For this review, use the dimensioned drawing (mm, ordinates from the lowest corner) and the shaded views. Coordinates: 2 decimals unless noted, no trailing zeros. Loops run counter-clockwise (first coordinate to the right, second up) from the corner with the lowest first, then second, coordinate; pieces in that order, holes last. Notation, with made-up numbers: (13.5, 48.25) -> (23.5, 48.25) arc R14 ccw to (23.5, 72.25) -> close; hole circle Ø11 at (-34.5, 7.25). An arc over 180 degrees is marked (long way). Use one line per item in the form item = value. Start each with the question number.
1. Consider section B-B (z = 13.3). State the section outline as (x, y) points.
2. For pin 1 (0.8 mm diameter, centred on x = 3.5, y = 1, fed in from -Z); pin 2 (4 mm diameter, centred on x = 15, z = 21.3, fed in from -Y); pin 3 (0.5 mm diameter, centred on y = 1, z = 4, fed in from -X), all flat-tipped, find the tip position at first contact; note any pin that passes through.
3. Consider section D-D (x = 19.5). State the section outline as (y, z) points.
4. Consider section C-C (y = 0.7). State how many separate pieces and enclosed holes the cut face has, then the cut area to 3 significant figures.
5. Consider section A-A (x = 15). State the section outline as (y, z) points.
6. Wall thickness on line 1 (Z direction, x = 15, y = 0.5); line 2 (X direction, y = 1.35, z = 13.3); line 3 (X direction, y = 0.9, z = 21.3): over which ranges is each line inside the solid? List them lowest first. Write a range as from..to.
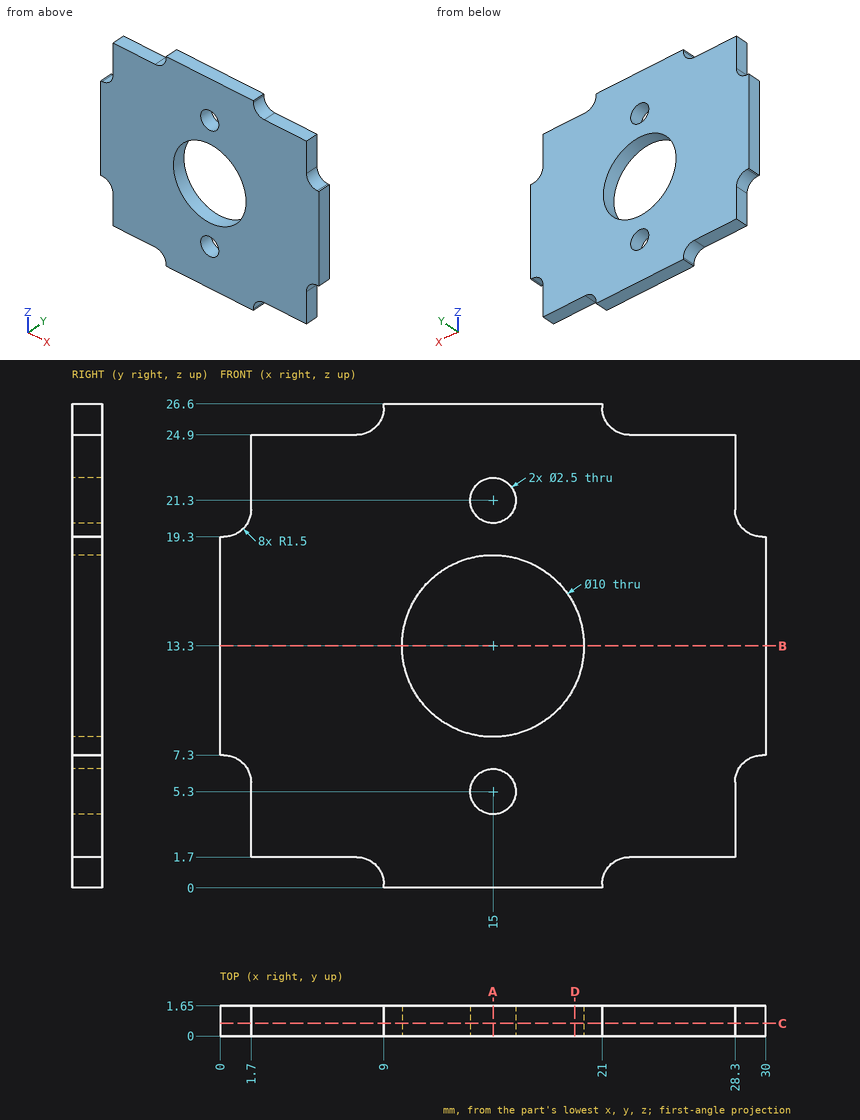
Geometry check:
q1.outline = (0, 0) -> (10, 0) -> (10, 1.65) -> (0, 1.65) -> close; (20, 0) -> (30, 0) -> (30, 1.65) -> (20, 1.65) -> close
q2.pin_1 = 1.7
q2.pin_2 = 0
q2.pin_3 = 1.7
q3.outline = (0, 0) -> (1.65, 0) -> (1.65, 11.12) -> (0, 11.12) -> close; (0, 15.48) -> (1.65, 15.48) -> (1.65, 26.6) -> (0, 26.6) -> close
q4.separate_pieces = 1
q4.enclosed_holes = 3
q4.area = 614 mm²
q5.outline = (0, 0) -> (1.65, 0) -> (1.65, 4.05) -> (0, 4.05) -> close; (0, 6.55) -> (1.65, 6.55) -> (1.65, 8.3) -> (0, 8.3) -> close; (0, 18.3) -> (1.65, 18.3) -> (1.65, 20.05) -> (0, 20.05) -> close; (0, 22.55) -> (1.65, 22.55) -> (1.65, 26.6) -> (0, 26.6) -> close
q6.line_1 = 0..4.05, 6.55..8.3, 18.3..20.05, 22.55..26.6
q6.line_2 = 0..10, 20..30
q6.line_3 = 1.7..13.75, 16.25..28.3
